Autodesk Inventor part; units mm, degrees
ref_plane "YZ Plane" through (0, 0, 0) normal (1, 0, 0) x (0, 1, 0)
ref_plane "XZ Plane" through (0, 0, 0) normal (0, 1, 0) x (-1, 0, 0)
ref_plane "XY Plane" through (0, 0, 0) normal (0, 0, 1) x (1, 0, 0)
sketch "スケッチ1" plane through (0, 0, 0) normal (0, 1, 0) x (-1, 0, 0)
  line L0 (16, -31) -> (16, 14)
  line L1 (16, 14) -> (-16, 14)
  line L2 (-16, 14) -> (-16, -31)
  line L3 (-16, -31) -> (16, -31)
  line L4 (0, 0) -> (0, -32.6995) construction
  point P0 (0, 14)
  dimension "d0" = 45
  dimension "d1" = 32
  dimension "d2" = 14
extrude "押し出し1" add sketch "スケッチ1" along normal blind 0.3
sketch "スケッチ4" plane through (0, 0.3, 0) normal (0, 1, 0) x (1, 0, 0)
  line L0 (0, 0) -> (-18.7084, 0) construction
  circle A0 centre (-6, 28.2) radius 1.7
  circle A1 centre (6, 28.2) radius 1.7
  line L1 (0, 0) -> (0, 29.6633) construction
  line L2 (16, 31) -> (-16, 31)
  point P0 (0, 31)
  dimension "d35" = 3.4
  dimension "d36" = 3.4
  dimension "d37" = 6
  dimension "d38" = 2.8
extrude "押し出し3" cut sketch "スケッチ4" against normal through all
sketch "スケッチ7" plane through (0, 0.3, 0) normal (0, 1, 0) x (1, 0, 0)
  circle A0 centre (-12.5, -10.4296) radius 1.7
  circle A1 centre (12.5, -10.4296) radius 1.7
  circle A2 centre (12.3554, 14.5704) radius 1.7
  circle A3 centre (-12.3554, 14.5704) radius 1.7
  line L0 (0, 0) -> (0, 34.4459) construction
  dimension "d47" = 3.4
  dimension "d48" = 3.4
  dimension "d49" = 3.4
  dimension "d50" = 3.4
  dimension "d51" = 25
  dimension "d52" = 25
extrude "押し出し6" cut sketch "スケッチ7" against normal through all
properties part number "B_holder_sub_muti-holes" material "ステンレス鋼 440C"
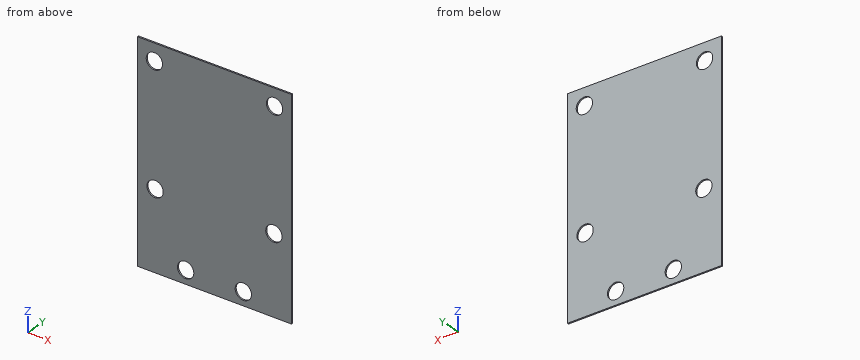
Geometry check sheet. Reference: the model listing, model coordinates, mm. Coordinates: 2 decimals unless noted, no trailing zeros. Loops run counter-clockwise (first coordinate to the right, second up) from the corner with the lowest first, then second, coordinate; pieces in that order, holes last.
Item 1: Sectioned sample at D-D, the plane x = -12.5. Record the boundary of the cut face in (y, z), then the cut area to 3 significant figures.
Item 2: Sectioned sample at C-C, the plane z = -27. Record the boundary of the cut face in (x, y).
Item 3: Thickness scan on line 1 (Z direction, x = -12.5, y = 0.15); line 2 (Z direction, x = 12, y = 0.1); line 3 (X direction, y = 0.1, z = -16). Record the ranges inside material, lowest first.
Item 4: Sectioned sample at B-B, the plane y = 0.25. Record the boundary of the cut face in (x, z), then the cut area to 3 significant figures.
Item 5: Sectioned sample at A-A, the plane x = -6. Record the boundary of the cut face in (y, z).
Check result:
1. outline: (0, -31) - (0.3, -31) - (0.3, -16.26) - (0, -16.26) - close; (0, -12.88) - (0.3, -12.88) - (0.3, 8.73) - (0, 8.73) - close; (0, 12.13) - (0.3, 12.13) - (0.3, 14) - (0, 14) - close
1. area: 11.5 mm2
2. outline: (-16, 0) - (-7.2, 0) - (-7.2, 0.3) - (-16, 0.3) - close; (-4.8, 0) - (4.8, 0) - (4.8, 0.3) - (-4.8, 0.3) - close; (7.2, 0) - (16, 0) - (16, 0.3) - (7.2, 0.3) - close
3. line 1: z = -31 to -16.26, -12.88 to 8.73, 12.13 to 14
3. line 2: z = -31 to -16.23, -12.91 to 8.8, 12.05 to 14
3. line 3: x = -16 to -13.28, -11.44 to 11.44, 13.28 to 16
4. outline: (-16, -31) - (16, -31) - (16, 14) - (-16, 14) - close; hole circle Ø3.4 at (-12.5, 10.43); hole circle Ø3.4 at (-12.36, -14.57); hole circle Ø3.4 at (-6, -28.2); hole circle Ø3.4 at (6, -28.2); hole circle Ø3.4 at (12.36, -14.57); hole circle Ø3.4 at (12.5, 10.43)
4. area: 1,390 mm2
5. outline: (0, -31) - (0.3, -31) - (0.3, -29.9) - (0, -29.9) - close; (0, -26.5) - (0.3, -26.5) - (0.3, 14) - (0, 14) - close
